Source: CAD feature listing. Evaluate the final solid. Frame: model axes, mm. A direction names the side the tool comes from. Give positions to 0.01 mm unless a question says otherwise; leave off trailing zeros. Write each loop counter-clockwise with the first axis right and the second up, starting at its lowest first coordinate (ties: lowest second). Pieces come first, ordered by that corner, then holes. Notation, with made-up numbers: M 17,75 L 23,75 A34 cw 23,114 Z; hole C 14,51 d5. An arc over 180 degrees is marked long. Use CSV: the item, a comma, the result in double quotes. Start each with the question number.
from build123d import *

# Parameters (mm, degrees)
SKETCH4_R           = 3.175
SKETCH4_R_2         = 3.96875
SKETCH4_R_3         = 5.1
SKETCH4_R_4         = 1.6
SKETCH4_R_5         = 2
BOSS_EXTRUDE2_DEPTH = 6.35


with BuildPart() as part:
    # Sketch4 → Boss-Extrude2 (new body)
    with BuildSketch(Plane(origin=(0, 0, 0), x_dir=(1, 0, 0), z_dir=(0, 1, 0))):
        with BuildLine():
            Line((41.886832424, -18.732457737), (20.296832424, -18.732457737))
            ThreePointArc((20.296832424, -18.732457737), (18.500781199, -17.988508961), (17.756832424, -16.192457737))
            Line((17.756832424, -16.192457737), (17.756832424, -16.158228087))
            ThreePointArc((17.756832424, -16.158228087), (17.384858036, -15.260202475), (16.486832424, -14.888228087))
            Line((16.486832424, -14.888228087), (10.176729358, -14.888228087))
            ThreePointArc((10.176729358, -14.888228087), (0.671575018, -18.021491142), (-9.04041606, -15.604359438))
            Line((-9.04041606, -15.604359438), (-15.242136468, -18.768748092))
            ThreePointArc((-15.242136468, -18.768748092), (-20.007104805, -18.207530981), (-21.312082241, -13.59050577))
            Line((-21.312082241, -13.59050577), (-12.82386942, 12.584286272))
            ThreePointArc((-12.82386942, 12.584286272), (-12.731158467, 12.971183794), (-12.7, 13.36781229))
            Line((-12.7, 13.36781229), (-12.7, 28.2575))
            ThreePointArc((-12.7, 28.2575), (-11.956051224, 30.053551224), (-10.16, 30.7975))
            Line((-10.16, 30.7975), (54.61, 30.7975))
            ThreePointArc((54.61, 30.7975), (56.406051224, 30.053551224), (57.15, 28.2575))
            Line((57.15, 28.2575), (57.15, 16.776257881))
            ThreePointArc((57.15, 16.776257881), (56.034076836, 14.082181045), (53.34, 12.966257881))
            Line((53.34, 12.966257881), (52.07, 12.966257881))
            ThreePointArc((52.07, 12.966257881), (49.375923164, 11.850334717), (48.26, 9.156257881))
            Line((48.26, 9.156257881), (48.26, -12.3825))
            ThreePointArc((48.26, -12.3825), (46.391929601, -16.880811578), (41.886832424, -18.732457737))
        make_face()
        with Locations(Location((0, 0, 0), (0, 0, 270))):
            Circle(SKETCH4_R, mode=Mode.SUBTRACT)
        with Locations(Location((-1.5875, 21.9075, 0), (0, 0, 270))):
            Circle(SKETCH4_R_2, mode=Mode.SUBTRACT)
        with Locations(Location((49.2125, 21.9075, 0), (0, 0, 270))):
            Circle(SKETCH4_R_2, mode=Mode.SUBTRACT)
        with Locations(Location((39.848481715, -4.1275, 0), (0, 0, 270))):
            Circle(SKETCH4_R_3, mode=Mode.SUBTRACT)
        with Locations(Location((39.848481715, -14.6275, 0), (0, 0, 270))):
            Circle(SKETCH4_R_4, mode=Mode.SUBTRACT)
        with Locations(Location((39.848481715, 6.3725, 0), (0, 0, 270))):
            Circle(SKETCH4_R_4, mode=Mode.SUBTRACT)
        with Locations(Location((24.012521227, -14.703599027, 0), (0, 0, 270))):
            Circle(SKETCH4_R_5, mode=Mode.SUBTRACT)
        with Locations(Location((-17.204660255, -14.9225, 0), (0, 0, 270))):
            Circle(SKETCH4_R_5, mode=Mode.SUBTRACT)
        with BuildLine():
            Line((40.81829921, 24.617647737), (16.8275, 10.766553356))
            ThreePointArc((16.8275, 10.766553356), (14.81487587, 10.537243801), (13.274563122, 11.852795168))
            Line((13.274563122, 11.852795168), (6.783830771, 25.160768644))
            ThreePointArc((6.783830771, 25.160768644), (6.848278127, 26.390497466), (7.92529921, 26.9875))
            Line((7.92529921, 26.9875), (40.18329921, 26.9875))
            ThreePointArc((40.18329921, 26.9875), (41.410025009, 26.046200187), (40.81829921, 24.617647737))
        make_face(mode=Mode.SUBTRACT)
        with BuildLine():
            Line((31.325699228, -2.62693366), (31.523640252, -0.070720194))
            ThreePointArc((31.523640252, -0.070720194), (30.334503757, 2.281113068), (27.699320049, 2.312291862))
            Line((27.699320049, 2.312291862), (15.869577834, -4.676031684))
            ThreePointArc((15.869577834, -4.676031684), (14.622916882, -6.777495975), (15.725443447, -8.958035098))
            Line((15.725443447, -8.958035098), (16.699675668, -9.625802289))
            ThreePointArc((16.699675668, -9.625802289), (17.939612893, -10.063131328), (19.232094548, -9.821900773))
            Line((19.232094548, -9.821900773), (29.889663519, -4.722023501))
            ThreePointArc((29.889663519, -4.722023501), (30.888370189, -3.866870885), (31.325699228, -2.62693366))
        make_face(mode=Mode.SUBTRACT)
        with BuildLine():
            Line((6.222926422, -4.3976797), (9.022181232, -8.938134359))
            ThreePointArc((9.022181232, -8.938134359), (-0.187421307, -12.698616982), (-9.282033212, -8.667978971))
            Line((-9.282033212, -8.667978971), (-6.35, -4.212113484))
            ThreePointArc((-6.35, -4.212113484), (-0.112452784, -7.619170189), (6.222926422, -4.3976797))
        make_face(mode=Mode.SUBTRACT)
    extrude(amount=-BOSS_EXTRUDE2_DEPTH)


solid = part.part
Item 1: Contact query for flat-ended pins moving along their axis: pin 1 Ø2 at (y, z) = (-1, 2) entering from +X; pin 2 Ø1.9 at (y, z) = (-3, -22.5) entering from -X; pin 3 Ø6.5 at (x, z) = (-1.59, -21.91) entering from -Y; pin 4 Ø1.9 at (x, y) = (14.5, -2.5) entering from +Z. Output: stop coordinate, or through.
Item 2: Section B-B (x = 0). State how many separate pieces and enclosed holes the cut face has, plus the area to 3 significant figures.
Item 3: Pull-direction query (Z, two-part tool) for faces 4 (the flat face through (57.15, -3, -23)), 5 (the flat face through (13, -3, 14.888)), 6 (the cylindrical face through (41.404, -3.131, -26.069)); classes: released by +Z, released by -Z, zero draft, split by the parting line, or undercut.
Item 4: Material intervals for probe 1 along X at (y, z) = (-4.25, 6.5); probe 2 along Z at (x, y) = (1.5, -2.5); probe 3 along Z at (x, y) = (40.5, -3.5), sorted ascending.
Item 5: Set-up query: faces 1 (the flat face through (-12.098, -3.131, 17.164)), 2 (the cylindrical face through (6.84, -3.13, -26.38)), 3 (the flat face through (48.26, -3, 1)). Return all of +Z, -Z, +X, -X, +Y, -Y with unobstructed straight access to the full face (end or side cutting, diameter ignored); none if empty.
Item 6: Section A-A (z = -21.5). Return the cut outline in (x, y), plus the area to 3 significant figures.
Output values:
1,pin 1,"stops at x = 48.26"
1,pin 2,"stops at x = -12.7"
1,pin 3,"passes through"
1,pin 4,"stops at z = 14.89"
2,separate pieces,"4"
2,enclosed holes,"0"
2,area,"191 mm2"
3,face 4,"zero draft"
3,face 5,"released by +Z"
3,face 6,"undercut"
4,probe 1,"x = -19.01 to -7.86, -3.98 to 3.98, 7.52 to 14.65, 26.17 to 35.33, 44.36 to 48.26"
4,probe 2,"z = -30.8 to -24.4, -19.41 to -2.8, 2.8 to 7.47, 12.61 to 17.97"
4,probe 3,"z = -30.8 to -26.95, -24.43 to -7.83, -4.91 to -0.93, 9.19 to 13.17, 16.09 to 18.73"
5,face 1,"+Z, +Y, -Y"
5,face 2,"+Y, -Y"
5,face 3,"+Z, +X, +Y, -Y"
6,outline,"M -12.7,-6.35 L -5.54,-6.35 L -5.54,0 L -12.7,0 Z; M 2.36,-6.35 L 8.57,-6.35 L 8.57,0 L 2.36,0 Z; M 35.42,-6.35 L 45.26,-6.35 L 45.26,0 L 35.42,0 Z; M 53.16,-6.35 L 57.15,-6.35 L 57.15,0 L 53.16,0 Z"
6,area,"173 mm2"
